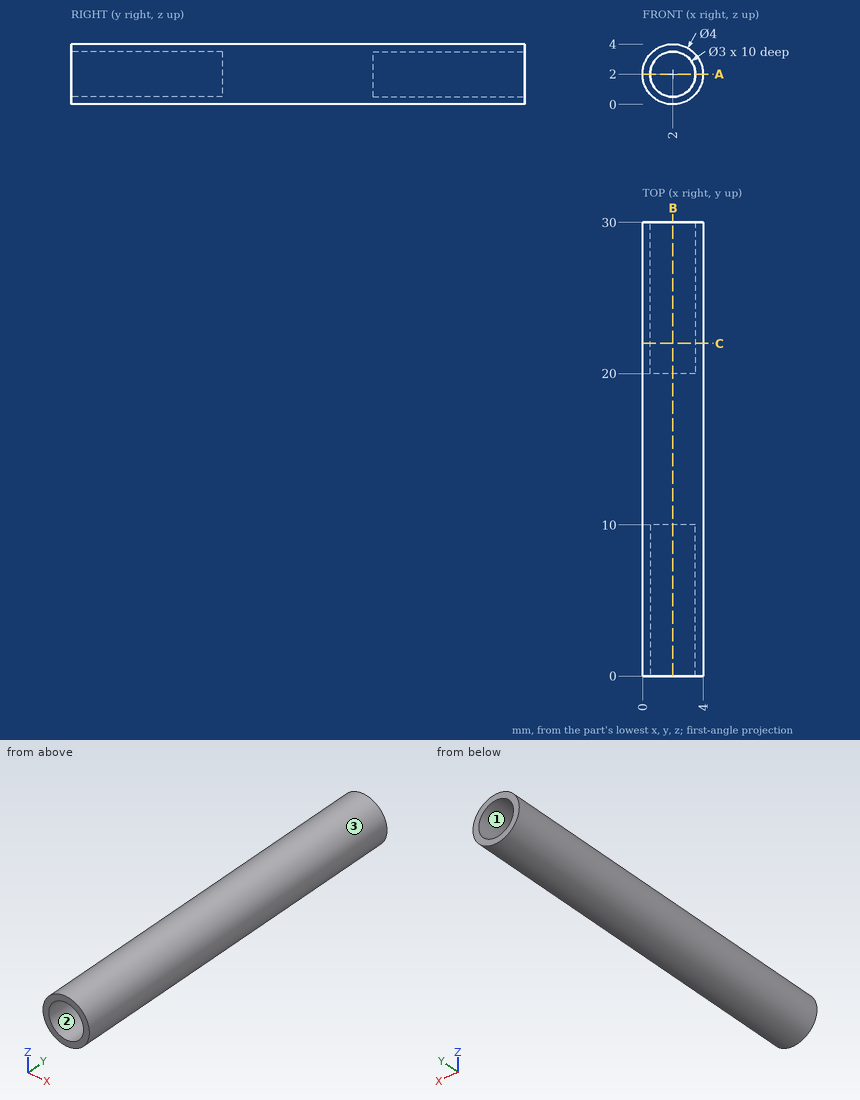
Check sheet for the drawn part. Datum: minimum x, y, z corner. Units: mm. Round coordinates to 2 decimals unless told otherwise and drop trailing zeros. Order: outer loops, then holes, each group sorted by start corner. A loop starts at its lowest first (then second) coordinate and runs counter-clockwise, first axis right, second up.
1. Thickness scan on L1, parallel to Z at x = 2, y = 5; L2, parallel to Y at x = 2.2, z = 3.4; L3, parallel to X at y = 3.5, z = 0.7. Record the ranges inside material, lowest first.
Final values:
L1: z = 0 to 0.5, 3.5 to 4
L2: y = 10 to 20
L3: x = 0.48 to 1.25, 2.75 to 3.52
2. Section check C-C on y = 22. Record the cut outline in (x, z), then the cut area to 3 significant figures.
Final values:
outline: circle Ø4 at (2, 2); hole circle Ø3 at (2, 2)
area: 5.50 mm2
3. Section check B-B on x = 2. Record the cut outline in (y, z).
Final values:
outline: (0, 0) - (30, 0) - (30, 0.5) - (20, 0.5) - (20, 3.5) - (30, 3.5) - (30, 4) - (0, 4) - (0, 3.5) - (10, 3.5) - (10, 0.5) - (0, 0.5) - close
4. Release check for a two-part mould opening along X. For the marked faces 1, 2 and 3 record: +X half, -X half, draft (parallel to the pull), parting line (faces both ways), or undercut.
Final values:
face 1: undercut
face 2: undercut
face 3: parting line
5. Go/stop test with a flat-tipped pin: P1, Ø1, axis at x = 1.5, z = 2.5, coming from the +Y side. Record where the tip stops, or that it passes through.
Final values:
P1: stops at y = 20
6. Section check A-A on z = 2. Record the cut outline in (x, y).
Final values:
outline: (0, 0) - (0.5, 0) - (0.5, 10) - (3.5, 10) - (3.5, 0) - (4, 0) - (4, 30) - (3.5, 30) - (3.5, 20) - (0.5, 20) - (0.5, 30) - (0, 30) - close
